The listing builds one solid part. Answer for the finished solid, in the listing's coordinates (mm). A direction names the side the tool comes from. Round coordinates to 2 decimals unless told otherwise and drop trailing zeros. Write each loop counter-clockwise with the first axis right and the second up, starting at its lowest first coordinate (ties: lowest second). Pieces come first, ordered by that corner, then holes.
Item 1: Find section C-C on z = -13. Give the vertices of the cut face in (x, y).
Item 2: Each of these flat-tipped pins is pushed along its axis until it touches: pin 1 (5 mm diameter, centred on x = 18, z = 13, fed in from +Y); pin 2 (6 mm diameter, centred on x = 0.5, z = 1, fed in from +Y); pin 3 (3 mm diameter, centred on x = 18, z = -13, fed in from -Y); pin 4 (5 mm diameter, centred on x = -19, z = -12.5, fed in from +Y). Where does it stop, or does it pass through?
Item 3: For a pull along Z with two mould halves and no side action, classify faces 5 (the face through (14.753, -7.395, 13.143)), 6 (the face through (23, -12, 0)), 7 (the face through (0, -12, -18)) as +Z half, -Z half, draft (parallel to the pull), parting line (faces both ways), or undercut.
Item 4: Find section D-D on x = 18. Give the vertices of the cut face in (y, z), then the cut area to 3 significant figures.
Item 5: Find the intervals of material crossed by probe 1 along Z at (x, y) = (18, -22.5); probe 2 along X at (y, z) = (-6.25, 13); probe 3 along Z at (x, y) = (-18, -21.5), in increasing order.
Item 6: A tool of negligible diameter and unlimited length cuts with its end or side. For faces 1 (the face through (4.203, -1.141, 7.126)), 2 (the face through (21.797, -12.325, -16.859)), 3 (the face through (-8, -14, 0)), 4 (the face through (-16.6, -15, -14.4)), from which of +Z, -Z, +X, -X, +Y, -Y can it reach the whole face along a straight path? Write none if from no direction.
Item 7: Find section A-A on x = -18. Give the vertices of the cut face in (y, z).
Item 8: Find section B-B on y = -18.5. Give the vertices of the cut face in (x, z).
```python
from build123d import *

# Parameters (mm, degrees)
F0_R         = 3.25
F0_R_2       = 1.6
F1_DEPTH     = 25
F2_DEPTH     = 15
F3_T1_DEPTH  = 24
F3_T3_DEPTH  = 22
F3_T5_DEPTH  = 14
F3_T7_DEPTH  = 26
F3_T9_DEPTH  = 31
F3_T11_DEPTH = 45
F3_S15_W     = 4
F3_S15_H     = 4
F3_T16_DEPTH = 4
F3_S21_W     = 4
F3_S21_H     = 4
F3_T22_DEPTH = 4
F3_T29_DEPTH = 32
F3_T33_DEPTH = 24


# Not quite as in the source:
# - a fillet or chamfer that OpenCascade refuses, or shapes differently, is made with other operations: its cross-section is extruded or revolved along the edge and cut away or added


with BuildPart() as f1:
    # F0 (on Front) → F1 (new body)
    with BuildSketch(Plane.XZ):
        Polygon((-23, 0), (-23, -18), (23, -18), (23, 18), (3, 18), (3, 0), align=None)
        with Locations((-18, -13)):
            Circle(F0_R, mode=Mode.SUBTRACT)
        with Locations((18, -13)):
            Circle(F0_R, mode=Mode.SUBTRACT)
        with Locations((18, 13)):
            Circle(F0_R, mode=Mode.SUBTRACT)
        with Locations((18, 13)):
            Circle(F0_R)
        with Locations((18, 13)):
            Circle(F0_R_2, mode=Mode.SUBTRACT)
        with Locations((18, -13)):
            Circle(F0_R)
        with Locations((18, -13)):
            Circle(F0_R_2, mode=Mode.SUBTRACT)
        with Locations((-18, -13)):
            Circle(F0_R)
        with Locations((-18, -13)):
            Circle(F0_R_2, mode=Mode.SUBTRACT)
    extrude(amount=F1_DEPTH)

    # F0 (on Front) → F2 (cut)
    with BuildSketch(Plane.XZ):
        with Locations((18, -13)):
            Circle(F0_R)
        with Locations((18, -13)):
            Circle(F0_R_2, mode=Mode.SUBTRACT)
        with Locations((-18, -13)):
            Circle(F0_R)
        with Locations((-18, -13)):
            Circle(F0_R_2, mode=Mode.SUBTRACT)
        with Locations((18, 13)):
            Circle(F0_R)
        with Locations((18, 13)):
            Circle(F0_R_2, mode=Mode.SUBTRACT)
    extrude(amount=F2_DEPTH, mode=Mode.SUBTRACT)

    # F3: fillet of radius 4 on 9 edges, made by hand

    # F3_s2 → F3_t1 (cut)
    with BuildSketch(Plane.XY.offset(-28)):
        with BuildLine():
            ThreePointArc((-23, -4), (-21.8284271247, -1.1715728753), (-19, 0))
            Line((-19, 0), (-23, 0))
            Line((-23, 0), (-23, -4))
        make_face()
    extrude(amount=F3_T1_DEPTH, mode=Mode.SUBTRACT)

    # F3_s4 → F3_t3 (cut)
    with BuildSketch(Plane.YZ.offset(-19)):
        with BuildLine():
            ThreePointArc((-4, 0), (-1.1715728753, -1.1715728753), (0, -4))
            Line((0, -4), (0, 0))
            Line((0, 0), (-4, 0))
        make_face()
    extrude(amount=F3_T3_DEPTH, mode=Mode.SUBTRACT)

    # F3_s6 → F3_t5 (cut)
    with BuildSketch(Plane.XY):
        with BuildLine():
            ThreePointArc((7, 0), (4.1715728753, -1.1715728753), (3, -4))
            Line((3, -4), (3, 0))
            Line((3, 0), (7, 0))
        make_face()
    extrude(amount=F3_T5_DEPTH, mode=Mode.SUBTRACT)

    # F3_s8 → F3_t7 (cut)
    with BuildSketch(Plane.YZ.offset(7)):
        with BuildLine():
            ThreePointArc((0, 14), (-1.1715728753, 16.8284271247), (-4, 18))
            Line((-4, 18), (0, 18))
            Line((0, 18), (0, 14))
        make_face()
    extrude(amount=F3_T7_DEPTH, mode=Mode.SUBTRACT)

    # F3_s10 → F3_t9 (cut)
    with BuildSketch(Plane.XZ.offset(4)):
        with BuildLine():
            ThreePointArc((-23, -4), (-21.8284271247, -1.1715728753), (-19, 0))
            Line((-19, 0), (-23, 0))
            Line((-23, 0), (-23, -4))
        make_face()
        with BuildLine():
            ThreePointArc((3, 14), (4.1715728753, 16.8284271247), (7, 18))
            Line((7, 18), (3, 18))
            Line((3, 18), (3, 14))
        make_face()
    extrude(amount=F3_T9_DEPTH, mode=Mode.SUBTRACT)

    # F3_s12 → F3_t11 (cut)
    with BuildSketch(Plane.XZ.offset(-10)):
        with BuildLine():
            ThreePointArc((-23, -14), (-21.8284271247, -16.8284271247), (-19, -18))
            Line((-19, -18), (-23, -18))
            Line((-23, -18), (-23, -14))
        make_face()
        with BuildLine():
            ThreePointArc((19, -18), (21.8284271247, -16.8284271247), (23, -14))
            Line((23, -14), (23, -18))
            Line((23, -18), (19, -18))
        make_face()
        with BuildLine():
            ThreePointArc((23, 14), (21.8284271247, 16.8284271247), (19, 18))
            Line((19, 18), (23, 18))
            Line((23, 18), (23, 14))
        make_face()
    extrude(amount=F3_T11_DEPTH, mode=Mode.SUBTRACT)


with BuildPart() as f3_tool14:
    # F3_s15 → F3_t16 (new body)
    with BuildSketch(Plane.YZ.offset(-19)):
        with Locations((-2, -2)):
            Rectangle(F3_S15_W, F3_S15_H)
    extrude(amount=-F3_T16_DEPTH)

    # F3_s17 → F3_t18 (revolve, cut)
    with BuildSketch(Plane(origin=(-19, -4, -4), x_dir=(0, -0.7071067812, -0.7071067812), z_dir=(0, 0.7071067812, -0.7071067812))):
        with BuildLine():
            ThreePointArc((0, -4), (4, 0), (0, 4))
            Line((0, 4), (0, -4))
        make_face()
    revolve(axis=Axis((-19, -4, -4), (-1, 0, 0)), mode=Mode.SUBTRACT)


with BuildPart() as f1_1:
    add(f1.part)

    # F3_t13: cut F3_tool14
    add(f3_tool14.part, mode=Mode.SUBTRACT)


with BuildPart() as f3_tool20:
    # F3_s21 → F3_t22 (new body)
    with BuildSketch(Plane.XZ.offset(4)):
        with Locations((5, 16)):
            Rectangle(F3_S21_W, F3_S21_H)
    extrude(amount=-F3_T22_DEPTH)

    # F3_s23 → F3_t24 (revolve, cut)
    with BuildSketch(Plane(origin=(7, -4, 14), x_dir=(0.7071067812, 0, -0.7071067812), z_dir=(0.7071067812, 0, 0.7071067812))):
        with BuildLine():
            ThreePointArc((0, -4), (4, 0), (0, 4))
            Line((0, 4), (0, -4))
        make_face()
    revolve(axis=Axis((7, -4, 14), (0, 1, 0)), mode=Mode.SUBTRACT)


with BuildPart() as f1_2:
    add(f1_1.part)

    # F3_t19: cut F3_tool20
    add(f3_tool20.part, mode=Mode.SUBTRACT)


with BuildPart() as f3_tool27:
    # F3_s28 → F3_t29 (new body)
    with BuildSketch(Plane.YZ.offset(13)):
        with BuildLine():
            ThreePointArc((-4, 0), (-1.1715728753, -1.1715728753), (0, -4))
            Line((0, -4), (0, 0))
            Line((0, 0), (-4, 0))
        make_face()
    extrude(amount=-F3_T29_DEPTH)

    split(bisect_by=Plane.YZ.offset(3), keep=Keep.TOP)


with BuildPart() as f3_tool31:
    # F3_s32 → F3_t33 (new body)
    with BuildSketch(Plane.XY.offset(14)):
        with BuildLine():
            ThreePointArc((7, 0), (4.1715728753, -1.1715728753), (3, -4))
            Line((3, -4), (3, 0))
            Line((3, 0), (7, 0))
        make_face()
    extrude(amount=-F3_T33_DEPTH)

    split(bisect_by=Plane.XY, keep=Keep.BOTTOM)


with BuildPart() as f3_tool27_1:
    add(f3_tool27.part)

    # F3_t35: intersect F3_tool31
    add(f3_tool31.part, mode=Mode.INTERSECT)


with BuildPart() as f1_3:
    add(f1_2.part)

    # F3_t25: cut F3_tool27
    add(f3_tool27_1.part, mode=Mode.SUBTRACT)


solid = f1_3.part
```
Check values:
1. outline: (-23, -25) - (-19.6, -25) - (-19.6, -15) - (-21.25, -15) - (-21.25, -0.69) arc R4 ccw to (-23, -4) - close; (-16.4, -25) - (16.4, -25) - (16.4, -15) - (14.75, -15) - (14.75, 0) - (-14.75, 0) - (-14.75, -15) - (-16.4, -15) - close; (19.6, -25) - (23, -25) - (23, 0) - (21.25, 0) - (21.25, -15) - (19.6, -15) - close
2. pin 1: stops at y = -15
2. pin 2: stops at y = -0.54
2. pin 3: passes through
2. pin 4: stops at y = -0.01
3. face 5: undercut
3. face 6: draft
3. face 7: -Z half
4. outline: (-25, -18) - (0, -18) - (0, -16.25) - (-15, -16.25) - (-15, -14.6) - (-25, -14.6) - close; (-25, -11.4) - (-15, -11.4) - (-15, -9.75) - (0, -9.75) - (0, 9.75) - (-15, 9.75) - (-15, 11.4) - (-25, 11.4) - close; (-25, 14.6) - (-15, 14.6) - (-15, 16.25) - (-0.69, 16.25) arc R4 ccw to (-4, 18) - (-25, 18) - close
4. area: 638 mm2
5. probe 1: z = -18 to -14.6, -11.4 to 11.4, 14.6 to 18
5. probe 2: x = 3 to 14.75, 21.25 to 23
5. probe 3: z = -18 to -14.6, -11.4 to 0
6. face 1: +Z, -X, +Y
6. face 2: -Z, +X, +Y, -Y
6. face 3: +Z, -X, +Y, -Y
6. face 4: +Y
7. outline: (-25, -18) - (0, -18) - (0, -16.25) - (-15, -16.25) - (-15, -14.6) - (-25, -14.6) - close; (-25, -11.4) - (-15, -11.4) - (-15, -9.75) - (0, -9.75) - (0, -4) arc R4 ccw to (-4, 0) - (-25, 0) - close
8. outline: (-23, -14) arc R4 ccw to (-19, -18) - (19, -18) arc R4 ccw to (23, -14) - (23, 14) arc R4 ccw to (19, 18) - (7, 18) arc R4 ccw to (3, 14) - (3, 0) - (-19, 0) arc R4 ccw to (-23, -4) - close; hole circle Ø3.2 at (-18, -13); hole circle Ø3.2 at (18, -13); hole circle Ø3.2 at (18, 13)
